Answer from the drawing. Dimensions are ordinates in mm from the lowest x, y and z of the part. Coordinates: 2 decimals unless noted, no trailing zeros. Loops run counter-clockwise (first coordinate to the right, second up) from the corner with the lowest first, then second, coordinate; pieces in that order, holes last. Notation, with made-up numbers: (36, 41) - (77, 41) arc R29 cw to (77, 76) - close; hole circle Ø1 at (87.25, 3.25). An arc over 180 degrees is marked (long way). Write each question's results on one line, items separated by ' | '. Start each with the question number.
1. A cutting plane is placed at C-C on z = 1.4. Determine the outline of the cut face in (x, y), then the cut area to 3 significant figures.
2. A cutting plane is placed at A-A on y = 7. Determine the outline of the cut face in (x, z).
3. Find the intervals of material crossed by line 1 along X through (y, z) = (13, 0.6); line 2 along Y through (x, z) = (47.75, 1.55); line 3 along X through (y, z) = (8.5, 1.7), in increasing order. Write a range as [from, to].
4. This flat-tipped pin is pushed along its axis until it touches: P1, Ø6, axis at x = 22, y = 9.5, coming from the +Z side. Where does it stop, or does it pass through?
5. A cutting plane is placed at B-B on x = 47.75. Determine the outline of the cut face in (y, z).
6. A cutting plane is placed at D-D on y = 13.25. Determine the outline of the cut face in (x, z).
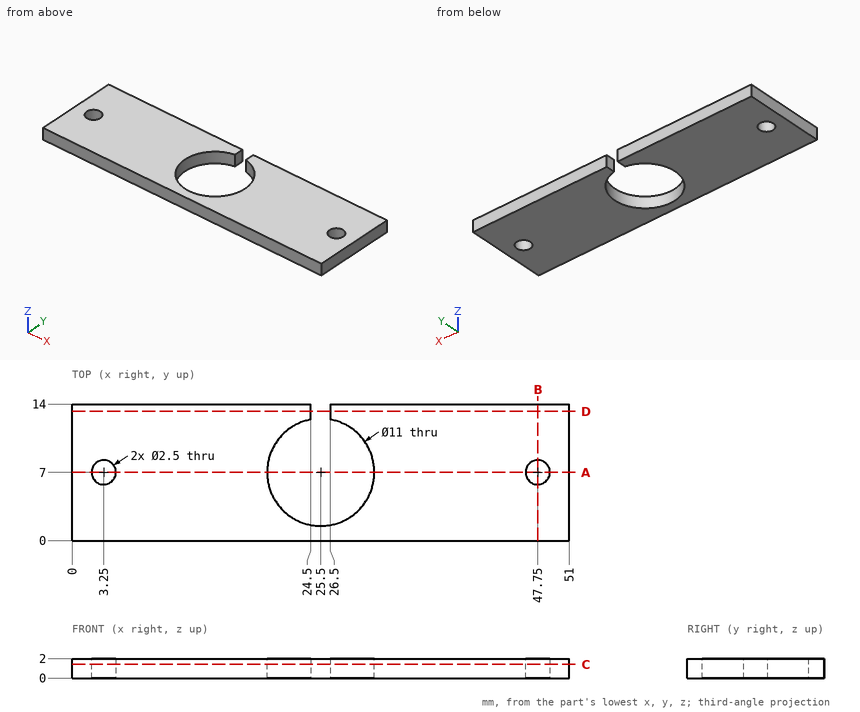
Values:
1) outline: (0, 0) - (51, 0) - (51, 14) - (26.5, 14) - (26.5, 12.41) arc R5.5 cw (long way) to (24.5, 12.41) - (24.5, 14) - (0, 14) - close; hole circle Ø2.5 at (3.25, 7); hole circle Ø2.5 at (47.75, 7) | area: 606 mm^2
2) outline: (0, 0) - (2, 0) - (2, 2) - (0, 2) - close; (4.5, 0) - (20, 0) - (20, 2) - (4.5, 2) - close; (31, 0) - (46.5, 0) - (46.5, 2) - (31, 2) - close; (49, 0) - (51, 0) - (51, 2) - (49, 2) - close
3) line 1: [0, 24.5], [26.5, 51] | line 2: [0, 5.75], [8.25, 14] | line 3: [0, 20.21], [30.79, 51]
4) P1: z = 2
5) outline: (0, 0) - (5.75, 0) - (5.75, 2) - (0, 2) - close; (8.25, 0) - (14, 0) - (14, 2) - (8.25, 2) - close
6) outline: (0, 0) - (24.5, 0) - (24.5, 2) - (0, 2) - close; (26.5, 0) - (51, 0) - (51, 2) - (26.5, 2) - close
